from build123d import *

# Parameters (mm, degrees)
F0_W     = 914.4
F0_H     = 393.7
F1_DEPTH = 25.4
F2_W     = 914.4
F2_H     = 31.75
F3_DEPTH = 12.7
F4_W     = 76.2
F4_H     = 304.8
F5_DEPTH = 38.1
F6_R     = 7.62
F7_R     = 5.07999


# Not quite as in the source:
# - a fillet or chamfer is up to 0.001 mm smaller than in the source, because OpenCascade refuses the exact size


with BuildPart() as f1:
    # F0 (on Top) → F1 (new body)
    with BuildSketch(Plane.XY):
        with Locations((457.2, 196.85)):
            Rectangle(F0_W, F0_H)
    extrude(amount=F1_DEPTH)

    # F2 (on face) → F3 (join)
    with BuildSketch(Plane.XY.offset(25.4)):
        with Locations((457.2, 377.825)):
            Rectangle(F2_W, F2_H)
        with Locations((457.2, 15.875)):
            Rectangle(F2_W, F2_H)
    extrude(amount=F3_DEPTH)

    # F4 (on face) → F5 (join)
    with BuildSketch(Plane.XY.offset(25.4)):
        with Locations((857.25, 196.85)):
            Rectangle(F4_W, F4_H)
    extrude(amount=F5_DEPTH)

    # F6
    f6_edges = [f1.edges().sort_by_distance(p)[0] for p in [
        (457.2, 393.7, 38.1),
        (457.2, 361.95, 38.1),
        (457.2, 31.75, 38.1),
        (457.2, 0, 38.1),
        (457.2, 393.7, 0),
        (457.2, 0, 0),
    ]]
    fillet(f6_edges, radius=F6_R)

    # F7 (radius 5.08 in the source; OpenCascade refuses exactly that, so slightly less here)
    f7_edges = [f1.edges().sort_by_distance(p)[0] for p in [
        (895.35, 196.85, 63.5),
        (857.25, 349.25, 63.5),
        (819.15, 196.85, 63.5),
        (857.25, 44.45, 63.5),
        (819.15, 44.45, 44.45),
        (895.35, 44.45, 44.45),
        (857.25, 44.45, 25.4),
        (457.2, 31.75, 25.4),
        (457.2, 361.95, 25.4),
        (914.4, 196.85, 25.4),
        (914.4, 393.7, 19.05),
        (914.4, 391.468154, 35.868154),
        (914.4, 391.468154, 2.231846),
        (914.4, 377.825, 38.1),
        (914.4, 196.85, 0),
        (914.4, 364.181846, 35.868154),
        (914.4, 2.231846, 2.231846),
        (914.4, 0, 19.05),
        (895.35, 196.85, 25.4),
        (819.15, 196.85, 25.4),
        (914.4, 2.231846, 35.868154),
        (914.4, 15.875, 38.1),
        (914.4, 29.518154, 35.868154),
    ]]
    fillet(f7_edges, radius=F7_R)


solid = f1.part
The listing builds one solid part. Answer for the finished solid, in the listing's coordinates (mm). A direction names the side the tool comes from. Give positions to 0.01 mm unless a question says otherwise; leave off trailing zeros. Loops run counter-clockwise (first coordinate to the right, second up) from the corner with the lowest first, then second, coordinate; pieces in that order, holes last. Notation, with made-up numbers: M 65,74.5 L 94,74.5 A25 cw 94,88.5 Z; hole C -12.75,-29 d3. An arc over 180 degrees is marked long. Answer as CSV lines item,"result".
Item 1: Given pin 1 Ø5 at (x, y) = (421.5, 374.5) entering from +Z; pin 2 Ø4 at (x, z) = (94.5, 36.5) entering from -Y; pin 3 Ø14 at (y, z) = (247, 39.5) entering from -X, each flat-ended and moving along its own axis, determine where each tip first touches the part or whether it passes through.
Values follow:
pin 1,"stops at z = 38.1"
pin 2,"stops at y = 1.15"
pin 3,"stops at x = 819.15"
Item 2: The part is cut by section B-B (y = 281). Give the vertices of the cut face in (x, z).
Values follow:
outline,"M 0,0 L 909.32,0 A5.08 ccw 914.4,5.08 L 914.4,20.32 A5.08 ccw 909.32,25.4 L 900.43,25.4 A5.08 cw 895.35,30.48 L 895.35,58.42 A5.08 ccw 890.27,63.5 L 824.23,63.5 A5.08 ccw 819.15,58.42 L 819.15,30.48 A5.08 cw 814.07,25.4 L 0,25.4 Z"
Item 3: Straight lines are drawn through the part: line 1 along Y through (x, z) = (865, 34); line 2 along Y through (x, z) = (471, 32); line 3 along Z through (x, y) = (352, 354.5). For each, find the intervals that lie inside material, in ascending order. Write a range as [from, to].
Values follow:
line 1,"y = [0.86, 30.89], [44.45, 349.25], [362.81, 392.84]"
line 2,"y = [0.15, 31.6], [362.1, 393.55]"
line 3,"z = [0, 25.4]"
Item 4: Which of the six approach directions +Z, -Z, +X, -X, +Y, -Y give full straight-line access (tool end or side, diameter ignored) to faces 1 (the flat face through (448, 199, 0)), 2 (the flat face through (895.35, 197, 44)), 3 (the flat face through (819.15, 197, 44)), 4 (the flat face through (857, 199, 63.5)), 5 (the flat face through (857, 349.25, 42))?
Values follow:
face 1,"-Z, +X, -X, +Y, -Y"
face 2,"+Z, +X"
face 3,"+Z, -X"
face 4,"+Z, +X, -X, +Y, -Y"
face 5,"+Z, +X, -X"
